from build123d import *

# Parameters (mm, degrees)
BOX002_W     = 10
BOX002_H     = 10
BOX002_DEPTH = 8
BOX001_W     = 2
BOX001_H     = 16
BOX001_DEPTH = 10
BOX_W        = 16
BOX_H        = 16
BOX_DEPTH    = 10


with BuildPart() as cube002:
    # Box002 → Box002 (new body)
    with BuildSketch(Plane(origin=(-5, -5, 0), x_dir=(1, 0, 0), z_dir=(0, 0, 1))):
        with Locations((5, 5)):
            Rectangle(BOX002_W, BOX002_H)
    extrude(amount=BOX002_DEPTH)


with BuildPart() as cube001:
    # Box001 → Box001 (new body)
    with BuildSketch(Plane(origin=(-1, -8, 10), x_dir=(1, 0, 0), z_dir=(0, 0, 1))):
        with Locations((1, 8)):
            Rectangle(BOX001_W, BOX001_H)
    extrude(amount=BOX001_DEPTH)


with BuildPart() as cut:
    # Box → Box (new body)
    with BuildSketch(Plane(origin=(-8, -8, 0), x_dir=(1, 0, 0), z_dir=(0, 0, 1))):
        with Locations((8, 8)):
            Rectangle(BOX_W, BOX_H)
    extrude(amount=BOX_DEPTH)

    # Fusion: union Cube001
    add(cube001.part)

    # Cut: cut Cube002
    add(cube002.part, mode=Mode.SUBTRACT)


solid = cut.part
Can you work these out from the model? Positions are in its coordinate system, mm. A direction names the side the tool comes from. Coordinates: 2 decimals unless noted, no trailing zeros. Write each loop counter-clockwise with the first axis right and the second up, starting at its lowest first coordinate (ties: lowest second). Pieces come first, ordered by that corner, then holes. Notation, with made-up numbers: (27.25, 50) -> (60.25, 50) arc R13 cw to (60.25, 59) -> close; hole circle Ø10 at (80.5, 56.5). An arc over 180 degrees is marked (long way). Write each question's results on one line, items separated by ' | '. Start each with the question number.
Q1. Imagine slicing it at A-A (z = 5). Write out the boundary of the cut face in (x, y).
Q2. Imagine slicing it at C-C (y = 3.75). Write out the boundary of the cut face in (x, z).
Q3. On a 3-axis mill with a long thin cutter (end or side, diameter ignored), from which of +Z, -Z, +X, -X, +Y, -Y can I reach the whole of each face in a straight line? I mean faces 5 (the face through (-5, 0, 4)), 6 (the face through (4, 0, 10)), 7 (the face through (-1, 0, 15)). Say none if no direction works.
Q4. Imagine slicing it at D-D (z = 15). Write out the boundary of the cut face in (x, y), then the cut area to 3 significant figures.
Q5. Imagine slicing it at B-B (x = 0). Write out the boundary of the cut face in (y, z), then the cut area to 3 significant figures.
Q6. I'm going to push flat-ended pins straight in: pin 1 (8 mm diameter, centred on x = -2.5, y = 2.5, fed in from -Z); pin 2 (5 mm diameter, centred on y = -3.5, z = 15.5, fed in from -X); pin 3 (2 mm diameter, centred on x = 4, y = -4, fed in from +Z); pin 4 (8 mm diameter, centred on y = -3.5, z = 14.5, fed in from +X). Where does each tip first touch, or does it pass through?
Q7. If I drill on probe 1 along X at (y, z) = (0.75, 7.5); probe 2 along Z at (x, y) = (-5, 5.5), over which ranges is the centre line in solid material (lowest first)?
Q8. We'd pull the mould along X, two halves only. Please class faces 1 (the face through (8, 0, 5)), 2 (the face through (-5, 0, 10)), 3 (the face through (0, 0, 8)), 4 (the face through (0, -5, 4)): +X half, -X half, draft (parallel to the pull), parting line (faces both ways), or undercut.
Taken from the geometry:
1) outline: (-8, -8) -> (8, -8) -> (8, 8) -> (-8, 8) -> close; hole (-5, -5) -> (5, -5) -> (5, 5) -> (-5, 5) -> close
2) outline: (-8, 0) -> (-5, 0) -> (-5, 8) -> (5, 8) -> (5, 0) -> (8, 0) -> (8, 10) -> (1, 10) -> (1, 20) -> (-1, 20) -> (-1, 10) -> (-8, 10) -> close
3) face 5: -Z | face 6: +Z, +X, +Y, -Y | face 7: +Z, -X, +Y, -Y
4) outline: (-1, -8) -> (1, -8) -> (1, 8) -> (-1, 8) -> close | area: 32.0 mm^2
5) outline: (-8, 0) -> (-5, 0) -> (-5, 8) -> (5, 8) -> (5, 0) -> (8, 0) -> (8, 20) -> (-8, 20) -> close | area: 240 mm^2
6) pin 1: stops at z = 0 | pin 2: stops at x = -1 | pin 3: stops at z = 10 | pin 4: stops at x = 1
7) probe 1: x = -8 to -5, 5 to 8 | probe 2: z = 0 to 10
8) face 1: +X half | face 2: draft | face 3: undercut | face 4: undercut
